Source: three-view drawing plus pictorial views. Frame: mm from the lowest corner of the part. Give positions to 0.01 mm unless a question says otherwise; leave off trailing zeros. Loops run counter-clockwise (first coordinate to the right, second up) from the corner with the lowest first, then second, coordinate; pieces in that order, holes last.
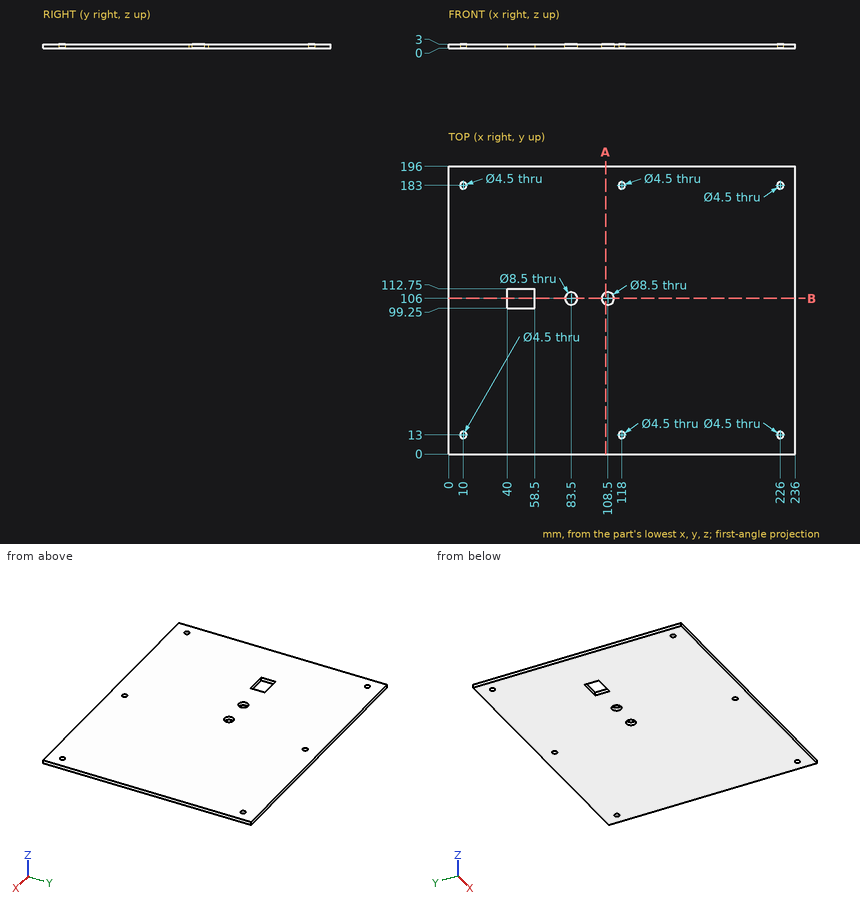
Q1. Section query B-B, the plane y = 106. Return loops of the section in (x, z), and give its area (4 significant figures).
Q2. Material intervals for probe 1 along X at (y, z) = (183, 1.25); probe 2 along Y at (x, z) = (226, 0.95), sorted ascending.
Q3. Section query A-A, the plane x = 107. Return loops of the section in (y, z), and give its area (3 significant figures).
Resolved:
1. outline: (0, 0) - (40, 0) - (40, 3) - (0, 3) - close; (58.5, 0) - (79.25, 0) - (79.25, 3) - (58.5, 3) - close; (87.75, 0) - (104.25, 0) - (104.25, 3) - (87.75, 3) - close; (112.75, 0) - (236, 0) - (236, 3) - (112.75, 3) - close
1. area: 601.5 mm2
2. probe 1: x = 0 to 7.75, 12.25 to 115.75, 120.25 to 223.75, 228.25 to 236
2. probe 2: y = 0 to 10.75, 15.25 to 180.75, 185.25 to 196
3. outline: (0, 0) - (102.02, 0) - (102.02, 3) - (0, 3) - close; (109.98, 0) - (196, 0) - (196, 3) - (109.98, 3) - close
3. area: 564 mm2
